Source: CAD feature listing. Evaluate the final solid. Frame: model axes, mm. A direction names the side the tool comes from. Round coordinates to 2 decimals unless told otherwise and drop trailing zeros. Order: outer loops, then holes, each group sorted by start corner. A loop starts at its lowest first (then second) coordinate and runs counter-clockwise, first axis right, second up. Notation, with made-up numbers: M -31.5,-39 L -10.5,-39 A17 ccw -10.5,-8 Z; hole C 20,-33 d5. An arc over 180 degrees is marked long. Answer as CSV lines item,"result". Start each with the question number.
Item 1: Section query C-C on y = -0.85. State how many separate pieces and enclosed holes the cut face has, plus the area to 3 significant figures.
Item 2: First-contact query: P1, Ø0.6, axis at y = -1, z = -5, coming from the -X side; P2, Ø1.4, axis at x = -1, y = -0.5, coming from the -Z side; P3, Ø0.6, axis at y = -1, z = -4.5, coming from the +X side. Flat tips, straight axial feed; report the tip coordinate or a pass-through.
Item 3: Section query A-A on z = 0. Return the cut outline in (x, y), plus the area to 3 significant figures.
Item 4: Line query: line 1 (Z direction, x = 0, y = -0.75); line 2 (Z direction, x = 0, y = 1.3); line 3 (Y direction, x = 2.75, z = -2.75). Output: solid intervals per line, ascending. Write a range as [from, to].
Item 5: Set-up query: faces 1 (the face through (-13.394, 0.465, -4.337)), 2 (the face through (10.6, -0.99, -3.34)). Return all of +Z, -Z, +X, -X, +Y, -Y with unobstructed straight access to the full face (end or side cutting, diameter ignored); none if empty.
Item 6: Section query B-B on x = 0.25. Return the cut outline in (y, z), plus the area to 3 significant figures.
Item 7: Pull-direction query (Z, two-part tool) for faces 3 (the face through (-11.636, 0.465, -5.941)), 4 (the face through (0.01, 0.46, 14.08)), 5 (the face through (-2.033, 0.465, -12.906)); classes: +Z half, -Z half, draft (parallel to the pull), parting line (faces both ways), or undercut.
Autodesk Inventor part; units mm, degrees
ref_plane "YZ Plane" through (0, 0, 0) normal (1, 0, 0) x (0, 1, 0)
ref_plane "XZ Plane" through (0, 0, 0) normal (0, 1, 0) x (-1, 0, 0)
ref_plane "XY Plane" through (0, 0, 0) normal (0, 0, 1) x (1, 0, 0)
sketch "Sketch1" plane through (0, 0, 0) normal (0, 1, 0) x (-1, 0, 0)
  circle A0 centre (0, 0) radius 1.5
  circle A1 centre (0, 0) radius 12.7
  dimension "d0" = 3
  dimension "d1" = 25.4
extrude "Extrusion1" add sketch "Sketch1" along normal blind 3
sketch "Sketch3" plane through (0, 0, 0) normal (0, -1, 0) x (1, 0, 0)
  circle A0 centre (0, 0) radius 11.1125
  circle A1 centre (0, 0) radius 12.7
  circle A2 centre (0, 0) radius 1.5
  circle A3 centre (0, 0) radius 12.7
  circle A4 centre (0, 0) radius 1.5
  circle A5 centre (0, 0) radius 12.7
  dimension "d14" = 22.225
extrude "Extrusion3" add sketch "Sketch3" along normal blind 2 contours A1
sketch "Sketch4" plane through (0, 0, 0) normal (0, -1, 0) x (1, 0, 0)
  circle A0 centre (0, 0) radius 1.5
  circle A1 centre (0, 0) radius 1.5
  line L0 (-1.4799, -0.2447) -> (-2.9799, -0.2447)
  line L1 (-2.9799, -0.2447) -> (-1.5, -0.2447)
  line L2 (-1.5, -0.2447) -> (-1.5, 7.3753)
  line L3 (-1.5, 7.3753) -> (-2.9799, 7.3753)
  line L4 (-2.9799, 7.3753) -> (-2.9799, -0.2447)
  line L5 (-2.9799, 7.3753) -> (-4.2499, 7.3753)
  line L6 (-4.2499, 7.3753) -> (-4.2499, 3.5653)
  line L7 (-4.2499, 3.5653) -> (-2.9799, 3.5653)
  line L8 (-2.9799, 3.5653) -> (-2.9799, 7.3753)
  line L9 (-1.5, 7.3753) -> (-0.23, 7.3753)
  line L10 (-0.23, 7.3753) -> (-0.23, 3.5653)
  line L11 (-0.23, 3.5653) -> (-1.5, 3.5653)
  line L12 (-1.5, 3.5653) -> (-1.5, 7.3753)
  line L13 (-2.9799, -0.2447) -> (-1.5, -0.2447)
  line L14 (-1.5, -0.2447) -> (-1.5, -7.2297)
  line L15 (-1.5, -7.2297) -> (-2.9799, -7.2297)
  line L16 (-2.9799, -7.2297) -> (-2.9799, -0.2447)
  line L17 (-2.9799, -7.2297) -> (-4.2499, -7.2297)
  line L18 (-4.2499, -7.2297) -> (-4.2499, -3.4197)
  line L19 (-4.2499, -3.4197) -> (-2.9799, -3.4197)
  line L20 (-2.9799, -3.4197) -> (-2.9799, -7.2297)
  line L21 (-1.5, -7.2297) -> (-0.23, -7.2297)
  line L22 (-0.23, -7.2297) -> (-0.23, -3.4197)
  line L23 (-0.23, -3.4197) -> (-1.5, -3.4197)
  line L24 (-1.5, -3.4197) -> (-1.5, -7.2297)
  line L25 (-2.9799, -7.2297) -> (-4.2499, -5.9597)
  line L26 (-2.9799, -7.2297) -> (-1.1839, -7.2297) construction
  point P0 (-2.9799, 3.5653)
  point P1 (-2.9799, -3.4197)
  dimension "d17" = 1.5
  dimension "d18" = 7.62
  dimension "d19" = 1.27
  dimension "d20" = 3.81
  dimension "d21" = 1.27
  dimension "d22" = 3.81
  dimension "d37" = 6.985
  dimension "d38" = 1.27
  dimension "d39" = 3.81
  dimension "d40" = 1.27
  dimension "d41" = 135
extrude "Extrusion4" add sketch "Sketch4" along normal blind 2 contours L23 L22 L21 L14 | L16 L25 L18 L19
sketch "Sketch5" plane through (0, 3, 0) normal (0, 1, 0) x (1, 0, 0)
  circle A0 centre (0, 0) radius 12.7
  circle A1 centre (0, 0) radius 1.5
  circle A2 centre (0, 0) radius 12.7
  line L0 (0, 12.7) -> (0, 14.605)
  line L1 (0, 14.605) -> (2.0758, 12.5292)
  line L2 (0, 14.605) -> (-2.0758, 12.5292)
  line L3 (0, 14.605) -> (2.9356, 14.605) construction
  line L4 (-4.5132, 13.8902) -> (-1.8975, 12.5574)
  line L5 (-3.9245, 12.0784) -> (-4.5132, 13.8902)
  line L6 (-4.5132, 13.8902) -> (-5.8459, 11.2745)
  line L7 (-8.5846, 11.8157) -> (-5.6851, 11.3565)
  line L8 (-7.4649, 10.2745) -> (-8.5846, 11.8157)
  line L9 (-8.5846, 11.8157) -> (-9.0438, 8.9162)
  line L10 (-11.8157, 8.5846) -> (-8.9162, 9.0438)
  line L11 (-10.2745, 7.4649) -> (-11.8157, 8.5846)
  line L12 (-11.8157, 8.5846) -> (-11.3565, 5.6851)
  line L13 (-13.8902, 4.5132) -> (-11.2745, 5.8459)
  line L14 (-12.0784, 3.9245) -> (-13.8902, 4.5132)
  line L15 (-13.8902, 4.5132) -> (-12.5574, 1.8975)
  line L16 (-14.605, 0) -> (-12.5292, 2.0758)
  line L17 (-12.7, 0) -> (-14.605, 0)
  line L18 (-14.605, 0) -> (-12.5292, -2.0758)
  line L19 (-13.8902, -4.5132) -> (-12.5574, -1.8975)
  line L20 (-12.0784, -3.9245) -> (-13.8902, -4.5132)
  line L21 (-13.8902, -4.5132) -> (-11.2745, -5.8459)
  line L22 (-11.8157, -8.5846) -> (-11.3565, -5.6851)
  line L23 (-10.2745, -7.4649) -> (-11.8157, -8.5846)
  line L24 (-11.8157, -8.5846) -> (-8.9162, -9.0438)
  line L25 (-8.5846, -11.8157) -> (-9.0438, -8.9162)
  line L26 (-7.4649, -10.2745) -> (-8.5846, -11.8157)
  line L27 (-8.5846, -11.8157) -> (-5.6851, -11.3565)
  line L28 (-4.5132, -13.8902) -> (-5.8459, -11.2745)
  line L29 (-3.9245, -12.0784) -> (-4.5132, -13.8902)
  line L30 (-4.5132, -13.8902) -> (-1.8975, -12.5574)
  line L31 (0, -14.605) -> (-2.0758, -12.5292)
  line L32 (0, -12.7) -> (0, -14.605)
  line L33 (0, -14.605) -> (2.0758, -12.5292)
  line L34 (4.5132, -13.8902) -> (1.8975, -12.5574)
  line L35 (3.9245, -12.0784) -> (4.5132, -13.8902)
  line L36 (4.5132, -13.8902) -> (5.8459, -11.2745)
  line L37 (8.5846, -11.8157) -> (5.6851, -11.3565)
  line L38 (7.4649, -10.2745) -> (8.5846, -11.8157)
  line L39 (8.5846, -11.8157) -> (9.0438, -8.9162)
  line L40 (11.8157, -8.5846) -> (8.9162, -9.0438)
  line L41 (10.2745, -7.4649) -> (11.8157, -8.5846)
  line L42 (11.8157, -8.5846) -> (11.3565, -5.6851)
  line L43 (13.8902, -4.5132) -> (11.2745, -5.8459)
  line L44 (12.0784, -3.9245) -> (13.8902, -4.5132)
  line L45 (13.8902, -4.5132) -> (12.5574, -1.8975)
  line L46 (14.605, 0) -> (12.5292, -2.0758)
  line L47 (12.7, 0) -> (14.605, 0)
  line L48 (14.605, 0) -> (12.5292, 2.0758)
  line L49 (13.8902, 4.5132) -> (12.5574, 1.8975)
  line L50 (12.0784, 3.9245) -> (13.8902, 4.5132)
  line L51 (13.8902, 4.5132) -> (11.2745, 5.8459)
  line L52 (11.8157, 8.5846) -> (11.3565, 5.6851)
  line L53 (10.2745, 7.4649) -> (11.8157, 8.5846)
  line L54 (11.8157, 8.5846) -> (8.9162, 9.0438)
  line L55 (8.5846, 11.8157) -> (9.0438, 8.9162)
  line L56 (7.4649, 10.2745) -> (8.5846, 11.8157)
  line L57 (8.5846, 11.8157) -> (5.6851, 11.3565)
  line L58 (4.5132, 13.8902) -> (5.8459, 11.2745)
  line L59 (3.9245, 12.0784) -> (4.5132, 13.8902)
  line L60 (4.5132, 13.8902) -> (1.8975, 12.5574)
  point P0 (-1.9969, 12.6081)
  point P1 (-5.7953, 11.3739)
  point P2 (-9.0264, 9.0264)
  point P3 (-11.3739, 5.7953)
  point P4 (-12.6081, 1.9969)
  point P5 (-12.6081, -1.9969)
  point P6 (-11.3739, -5.7953)
  point P7 (-9.0264, -9.0264)
  point P8 (-5.7953, -11.3739)
  point P9 (-1.9969, -12.6081)
  point P10 (1.9969, -12.6081)
  point P11 (5.7953, -11.3739)
  point P12 (9.0264, -9.0264)
  point P13 (11.3739, -5.7953)
  point P14 (12.6081, -1.9969)
  point P15 (12.6081, 1.9969)
  point P16 (11.3739, 5.7953)
  point P17 (9.0264, 9.0264)
  point P18 (5.7953, 11.3739)
  point P19 (1.9969, 12.6081)
  dimension "d28" = 1.905
  dimension "d29" = 45
  dimension "d30" = 135
  dimension "d33" = 360
extrude "Extrusion5" add sketch "Sketch5" against normal up to surface (5 mm away) contours L47 L46 L45 A0 | A0 L49 L48 L47 | A0 L48 L49 | L45 L46 A0 | A0 L50 L49 L48 | L46 L45 L44 A0 | A0 L52 L51 L50 | L44 L43 L42 A0 | A0 L51 L52 | L51 A0 L53 L52 | L42 L43 A0 | L42 L41 A0 L43 | L53 A0 L55 L54 | L40 L39 A0 L41 | L55 A0 L54 | L54 A0 L56 L55 | L40 A0 L39 | L39 L38 A0 L40 | L56 A0 L58 L57 | L37 L36 A0 L38 | L58 A0 L57 | L57 A0 L59 L58 | L37 A0 L36 | L36 L35 A0 L37 | L59 A0 L1 L60 | L34 L33 A0 L35 | L60 A0 L0 L1 | L1 A0 L60 | L34 A0 L33 | L33 L32 A0 L34 | L0 A0 L4 L2 | L31 L30 A0 L32 | L4 A0 L2 | L2 A0 L5 L4 | L31 A0 L30 | L30 L29 A0 L31 | L5 A0 L7 L6 | L28 L27 A0 L29 | L7 A0 L6 | L6 A0 L8 L7 | L28 A0 L27 | L27 L26 A0 L28 | L8 A0 L10 L9 | L25 L24 A0 L26 | L10 A0 L9 | L9 A0 L11 L10 | L25 A0 L24 | L24 L23 A0 L25 | L11 A0 L13 L12 | L22 L21 A0 L23 | L13 A0 L12 | L12 A0 L14 L13 | L22 A0 L21 | L21 L20 A0 L22 | L14 A0 L16 L15 | L19 L18 A0 L20 | L16 A0 L15 | L15 A0 L17 L16 | L19 A0 L18 | L18 L17 A0 L19
fillet "Fillet1" radius 1.27 40 edges at (11.8157, 0.5, 8.5846) (8.5846, 0.5, 11.8157) (4.5132, 0.5, 13.8902) (0, 0.5, 14.605) (-4.5132, 0.5, 13.8902) (-8.5846, 0.5, 11.8157) (-11.8157, 0.5, 8.5846) (-13.8902, 0.5, 4.5132) (-14.605, 0.5, 0) (-13.8902, 0.5, -4.5132) (-11.8157, 0.5, -8.5846) (-8.5846, 0.5, -11.8157) (-4.5132, 0.5, -13.8902) (0, 0.5, -14.605) (4.5132, 0.5, -13.8902) (8.5846, 0.5, -11.8157) (11.8157, 0.5, -8.5846) (9.0264, 0.5, -9.0264) (13.8902, 0.5, -4.5132) (14.605, 0.5, 0) (13.8902, 0.5, 4.5132) (11.3739, 0.5, -5.7953) (12.6081, 0.5, -1.9969) (12.6081, 0.5, 1.9969) (11.3739, 0.5, 5.7953) (9.0264, 0.5, 9.0264) (5.7953, 0.5, 11.3739) (1.9969, 0.5, 12.6081) (-1.9969, 0.5, 12.6081) (-5.7953, 0.5, 11.3739) (-9.0264, 0.5, 9.0264) (-11.3739, 0.5, 5.7953) (-12.6081, 0.5, 1.9969) (-12.6081, 0.5, -1.9969) (-11.3739, 0.5, -5.7953) (-9.0264, 0.5, -9.0264) (-5.7953, 0.5, -11.3739) (-1.9969, 0.5, -12.6081) (1.9969, 0.5, -12.6081) (5.7953, 0.5, -11.3739)
properties part number "Knob"
Results:
1,separate pieces,"3"
1,enclosed holes,"1"
1,area,"200 mm^2"
2,P1,"x = -13.21"
2,P2,"z = -14.04"
2,P3,"x = 13.43"
3,outline,"M -14.08,-2 L -11.11,-2 L -11.11,0 L -1.5,0 L -1.5,3 L -14.08,3 Z; M 1.5,0 L 11.11,0 L 11.11,-2 L 14.08,-2 L 14.08,3 L 1.5,3 Z"
3,area,"87.3 mm^2"
4,line 1,"[-14.08, -11.11], [11.11, 14.08]"
4,line 2,"[-14.08, -1.5], [1.5, 14.08]"
4,line 3,"[0, 3]"
5,face 1,"-X, +Y, -Y"
5,face 2,"-Y"
6,outline,"M -2,-14.05 L 3,-14.05 L 3,-1.48 L 0,-1.48 L 0,-11.11 L -2,-11.11 Z; M -2,11.11 L 0,11.11 L 0,1.48 L 3,1.48 L 3,14.05 L -2,14.05 Z"
6,area,"87.2 mm^2"
7,face 3,"undercut"
7,face 4,"+Z half"
7,face 5,"-Z half"
